Source: CAD feature listing. Evaluate the final solid. Frame: model axes, mm. Give positions to 0.01 mm unless a question says otherwise; leave off trailing zeros. Loops run counter-clockwise (first coordinate to the right, second up) from the corner with the lowest first, then second, coordinate; pieces in that order, holes last. Notation, with made-up numbers: (55.5, 31.5) -> (90.5, 31.5) arc R28 cw to (90.5, 53.5) -> close; hole circle Ø11 at (27.5, 48.5). An arc over 180 degrees is marked (long way). Put each result on its own line as item: value.
```python
from build123d import *

# Parameters (mm, degrees)
SKETCH1_W           = 158
SKETCH1_H           = 55
BOSS_EXTRUDE1_DEPTH = 4
CUT_EXTRUDE2_REACH  = 169.347
SKETCH2_R           = 1.5


with BuildPart() as part:
    # Sketch1 → Boss-Extrude1 (new body)
    with BuildSketch(Plane(origin=(0, 0, 0), x_dir=(1, 0, 0), z_dir=(0, 1, 0))):
        with Locations((79, 27.5)):
            Rectangle(SKETCH1_W, SKETCH1_H)
    extrude(amount=BOSS_EXTRUDE1_DEPTH)

    # Sketch2 → Cut-Extrude2 (cut, up to next)
    with BuildSketch(Plane(origin=(0, 4, 0), x_dir=(1, 0, 0), z_dir=(0, 1, 0)), mode=Mode.PRIVATE) as cut_extrude2_sk1:
        with Locations(Location((110.75, 36.39, 0), (0, 0, 270))):
            Circle(SKETCH2_R)
    cut_extrude2_tool1 = extrude(cut_extrude2_sk1.sketch, amount=-CUT_EXTRUDE2_REACH, mode=Mode.PRIVATE) & part.part
    # Sketch2 → Cut-Extrude2 (cut, up to next)
    with BuildSketch(Plane(origin=(0, 4, 0), x_dir=(1, 0, 0), z_dir=(0, 1, 0)), mode=Mode.PRIVATE) as cut_extrude2_sk2:
        with Locations(Location((59.95, 51.63, 0), (0, 0, 270))):
            Circle(SKETCH2_R)
    cut_extrude2_tool2 = extrude(cut_extrude2_sk2.sketch, amount=-CUT_EXTRUDE2_REACH, mode=Mode.PRIVATE) & part.part
    # Sketch2 → Cut-Extrude2 (cut, up to next)
    with BuildSketch(Plane(origin=(0, 4, 0), x_dir=(1, 0, 0), z_dir=(0, 1, 0)), mode=Mode.PRIVATE) as cut_extrude2_sk3:
        with Locations(Location((110.75, 8.45, 0), (0, 0, 270))):
            Circle(SKETCH2_R)
    cut_extrude2_tool3 = extrude(cut_extrude2_sk3.sketch, amount=-CUT_EXTRUDE2_REACH, mode=Mode.PRIVATE) & part.part
    # Sketch2 → Cut-Extrude2 (cut, up to next)
    with BuildSketch(Plane(origin=(0, 4, 0), x_dir=(1, 0, 0), z_dir=(0, 1, 0)), mode=Mode.PRIVATE) as cut_extrude2_sk4:
        with Locations(Location((58.68, 3.37, 0), (0, 0, 270))):
            Circle(SKETCH2_R)
    cut_extrude2_tool4 = extrude(cut_extrude2_sk4.sketch, amount=-CUT_EXTRUDE2_REACH, mode=Mode.PRIVATE) & part.part
    add(cut_extrude2_tool1.solids().sort_by_distance((110.75, 4, -36.39))[0], mode=Mode.SUBTRACT)
    add(cut_extrude2_tool2.solids().sort_by_distance((59.95, 4, -51.63))[0], mode=Mode.SUBTRACT)
    add(cut_extrude2_tool3.solids().sort_by_distance((110.75, 4, -8.45))[0], mode=Mode.SUBTRACT)
    add(cut_extrude2_tool4.solids().sort_by_distance((58.68, 4, -3.37))[0], mode=Mode.SUBTRACT)


solid = part.part
```
(1) Section A-A on x = 110.75. Return loops of the section in (y, z).
Calculated:
outline: (0, -55) -> (4, -55) -> (4, -37.89) -> (0, -37.89) -> close; (0, -34.89) -> (4, -34.89) -> (4, -9.95) -> (0, -9.95) -> close; (0, -6.95) -> (4, -6.95) -> (4, 0) -> (0, 0) -> close
(2) Line query: probe 1 along Z at (x, y) = (110.75, 2.1); probe 2 along X at (y, z) = (0.95, -3.37); probe 3 along X at (y, z) = (3.05, -8.5). Output: solid intervals per line, ascending. Write a range as from..to.
Calculated:
probe 1: z = -55..-37.89, -34.89..-9.95, -6.95..0
probe 2: x = 0..57.18, 60.18..158
probe 3: x = 0..109.25, 112.25..158
(3) Draft query along X for faces 1 (the flat face through (158, 2, -27)), 2 (the flat face through (78, 4, -28)), 3 (the cylindrical face through (61, 2, -52.7)). Return one class per face: released by +X, released by -X, zero draft, split by the parting line, or undercut.
Calculated:
face 1: released by +X
face 2: zero draft
face 3: undercut
(4) Section B-B on z = -8.45. Return loops of the section in (x, y), then the cut area to 3 significant figures.
Calculated:
outline: (0, 0) -> (109.25, 0) -> (109.25, 4) -> (0, 4) -> close; (112.25, 0) -> (158, 0) -> (158, 4) -> (112.25, 4) -> close
area: 620 mm²
